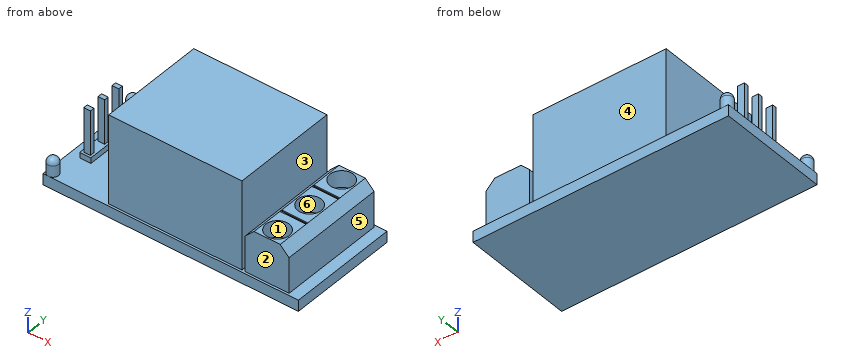
```python
from build123d import *

# Parameters (mm, degrees)
SKETCH1_W           = 23
SKETCH1_H           = 10
BOSS_EXTRUDE1_DEPTH = 1
SKETCH2_W           = 3.95
SKETCH2_H           = 9.6
BOSS_EXTRUDE2_DEPTH = 4
SKETCH5_W           = 12
SKETCH5_H           = 9.6
BOSS_EXTRUDE3_DEPTH = 8
CUT_EXTRUDE1_REACH  = 28.571
SKETCH7_R           = 1.05
CUT_EXTRUDE3_DEPTH  = 1.5
SKETCH9_W           = 2.35
SKETCH9_H           = 0.2
CUT_EXTRUDE4_DEPTH  = 0.1
SKETCH10_W          = 1
SKETCH10_H          = 4
BOSS_EXTRUDE4_DEPTH = 0.5
SKETCH11_W          = 0.6
SKETCH11_H          = 0.4
BOSS_EXTRUDE5_DEPTH = 4
SKETCH12_R          = 0.5
BOSS_EXTRUDE6_DEPTH = 1.5
FILLET3_R           = 0.5


with BuildPart() as part:
    # Sketch1 → Boss-Extrude1 (new body)
    with BuildSketch(Plane.XY):
        with Locations((11.5, -5)):
            Rectangle(SKETCH1_W, SKETCH1_H)
    extrude(amount=BOSS_EXTRUDE1_DEPTH)

    # Sketch2 → Boss-Extrude2 (add)
    with BuildSketch(Plane.XY.offset(1)):
        with Locations((20.025, -5)):
            Rectangle(SKETCH2_W, SKETCH2_H)
    extrude(amount=BOSS_EXTRUDE2_DEPTH)

    # Sketch5 → Boss-Extrude3 (add)
    with BuildSketch(Plane.XY.offset(1)):
        with Locations((11.757840523, -5)):
            Rectangle(SKETCH5_W, SKETCH5_H)
    extrude(amount=BOSS_EXTRUDE3_DEPTH)

    # Sketch6 → Cut-Extrude1 (cut, up to next)
    with BuildSketch(Plane.XZ.offset(9.8), mode=Mode.PRIVATE) as cut_extrude1_sk1:
        Polygon((21.2, 5), (22, 4.2), (22, 5), align=None)
    cut_extrude1_tool1 = extrude(cut_extrude1_sk1.sketch, amount=-CUT_EXTRUDE1_REACH, mode=Mode.PRIVATE) & part.part
    # Sketch6 → Cut-Extrude1 (cut, up to next)
    with BuildSketch(Plane.XZ.offset(9.8), mode=Mode.PRIVATE) as cut_extrude1_sk2:
        Polygon((18.05, 5), (18.85, 5), (18.05, 4.2), align=None)
    cut_extrude1_tool2 = extrude(cut_extrude1_sk2.sketch, amount=-CUT_EXTRUDE1_REACH, mode=Mode.PRIVATE) & part.part
    add(cut_extrude1_tool1.solids().sort_by_distance((21.733333, -9.8, 4.733333))[0], mode=Mode.SUBTRACT)
    add(cut_extrude1_tool2.solids().sort_by_distance((18.316667, -9.8, 4.733333))[0], mode=Mode.SUBTRACT)

    # Sketch7 → Cut-Extrude3 (cut)
    with BuildSketch(Plane.XY.offset(5)):
        with Locations((20.025, -8.625)):
            Circle(SKETCH7_R)
        with Locations((20.025, -5.005)):
            Circle(SKETCH7_R)
        with Locations((20.025, -1.385)):
            Circle(SKETCH7_R)
    extrude(amount=-CUT_EXTRUDE3_DEPTH, mode=Mode.SUBTRACT)

    # Sketch9 → Cut-Extrude4 (cut)
    with BuildSketch(Plane.XY.offset(5)):
        with Locations((20.025, -6.783672737)):
            Rectangle(SKETCH9_W, SKETCH9_H)
        with Locations((20.025, -3.163989789)):
            Rectangle(SKETCH9_W, SKETCH9_H)
    extrude(amount=-CUT_EXTRUDE4_DEPTH, mode=Mode.SUBTRACT)

    # Sketch10 → Boss-Extrude4 (add)
    with BuildSketch(Plane.XY.offset(1)):
        with Locations((1.418300491, -5)):
            Rectangle(SKETCH10_W, SKETCH10_H)
    extrude(amount=BOSS_EXTRUDE4_DEPTH)

    # Sketch11 → Boss-Extrude5 (add)
    with BuildSketch(Plane.XY.offset(1.5)):
        with Locations((1.418300491, -5)):
            Rectangle(SKETCH11_W, SKETCH11_H)
        with Locations((1.418300491, -3.4)):
            Rectangle(SKETCH11_W, SKETCH11_H)
        with Locations((1.418300491, -6.6)):
            Rectangle(SKETCH11_W, SKETCH11_H)
    extrude(amount=BOSS_EXTRUDE5_DEPTH)

    # Sketch12 → Boss-Extrude6 (add)
    with BuildSketch(Plane.XY.offset(1)):
        with Locations(Location((0.5, -9.5, 0), (0, 0, 180))):
            Circle(SKETCH12_R)
        with Locations(Location((0.5, -0.5, 0), (0, 0, 180))):
            Circle(SKETCH12_R)
    extrude(amount=BOSS_EXTRUDE6_DEPTH)

    # Fillet3
    fillet3_edges = [part.edges().sort_by_distance(p)[0] for p in [
        (1, -0.5, 2.5),
        (1, -9.5, 2.5),
    ]]
    fillet(fillet3_edges, radius=FILLET3_R)


solid = part.part
```
Design review of the part built by this model. Coordinates are the model's own, in mm. Face numbers are marked on the shaded views. A direction names the side the tool comes from. Coordinates: 2 decimals unless noted, no trailing zeros. Order: outer loops, then holes, each group sorted by start corner. A loop starts at its lowest first (then second) coordinate and runs counter-clockwise, first axis right, second up.
1) Take a section at B-B, the plane y = -7.25. Give the boundary of the cut face in (x, z).
2) Mouldability with a two-part tool opening along X and no side actions: class the marked faces 4, 5 and 6 as +X half, -X half, draft (parallel to the pull), parting line (faces both ways), or undercut.
3) Wall thickness on line 1 along X through (y, z) = (-6.25, 2.5); line 2 along X through (y, z) = (-5.5, 3.75); line 3 along Z through (x, y) = (20.25, -4.75): over which ranges is each line inside the solid? List them lowest first.
4) For the marked faces 1, 2 and 3, list the 3-axis set-ups (+Z, -Z, +X, -X, +Y, -Y) from which the entire face can be reached by the end or side of a thin tool; tool diameter is ignored.
5) Take a section at A-A, the plane z = 1.75. Give the boundary of the cut face in (x, y), and give its area (3 significant figures).
6) Take a section at D-D, the plane z = 7. Give the boundary of the cut face in (x, y).
7) Take a section at C-C, the plane x = 15.25. Give the boundary of the cut face in (y, z), and give its area (3 significant figures).
8) Clearance check with flat-ended pins moving along their axes: pin 1 (0.7 mm diameter, centred on x = 1.5, z = 3.5, fed in from -Y); pin 2 (2.5 mm diameter, centred on x = 12.5, z = 4.5, fed in from +Y); pin 3 (1 mm diameter, centred on y = -6.5, z = 2.5, fed in from +X). State where each tip first meets the part, or that it passes through.
Returned:
1. outline: (0, 0) - (23, 0) - (23, 1) - (22, 1) - (22, 4.2) - (21.2, 5) - (18.85, 5) - (18.05, 4.2) - (18.05, 1) - (17.76, 1) - (17.76, 9) - (5.76, 9) - (5.76, 1) - (0, 1) - close
2. face 4: draft
2. face 5: +X half
2. face 6: undercut
3. line 1: x = 5.76 to 17.76, 18.05 to 22
3. line 2: x = 5.76 to 17.76, 18.05 to 19.1, 20.95 to 22
3. line 3: z = 0 to 3.5
4. face 1: +Z
4. face 2: +Z, +X, -Y
4. face 3: +Z, +Y, -Y
5. outline: circle Ø1 at (0.5, -9.5); circle Ø1 at (0.5, -0.5); (1.12, -6.8) - (1.72, -6.8) - (1.72, -6.4) - (1.12, -6.4) - close; (1.12, -5.2) - (1.72, -5.2) - (1.72, -4.8) - (1.12, -4.8) - close; (1.12, -3.6) - (1.72, -3.6) - (1.72, -3.2) - (1.12, -3.2) - close; (5.76, -9.8) - (17.76, -9.8) - (17.76, -0.2) - (5.76, -0.2) - close; (18.05, -9.8) - (22, -9.8) - (22, -0.2) - (18.05, -0.2) - close
5. area: 155 mm2
6. outline: (5.76, -9.8) - (17.76, -9.8) - (17.76, -0.2) - (5.76, -0.2) - close
7. outline: (-10, 0) - (0, 0) - (0, 1) - (-0.2, 1) - (-0.2, 9) - (-9.8, 9) - (-9.8, 1) - (-10, 1) - close
7. area: 86.8 mm2
8. pin 1: stops at y = -6.8
8. pin 2: stops at y = -0.2
8. pin 3: stops at x = 22
